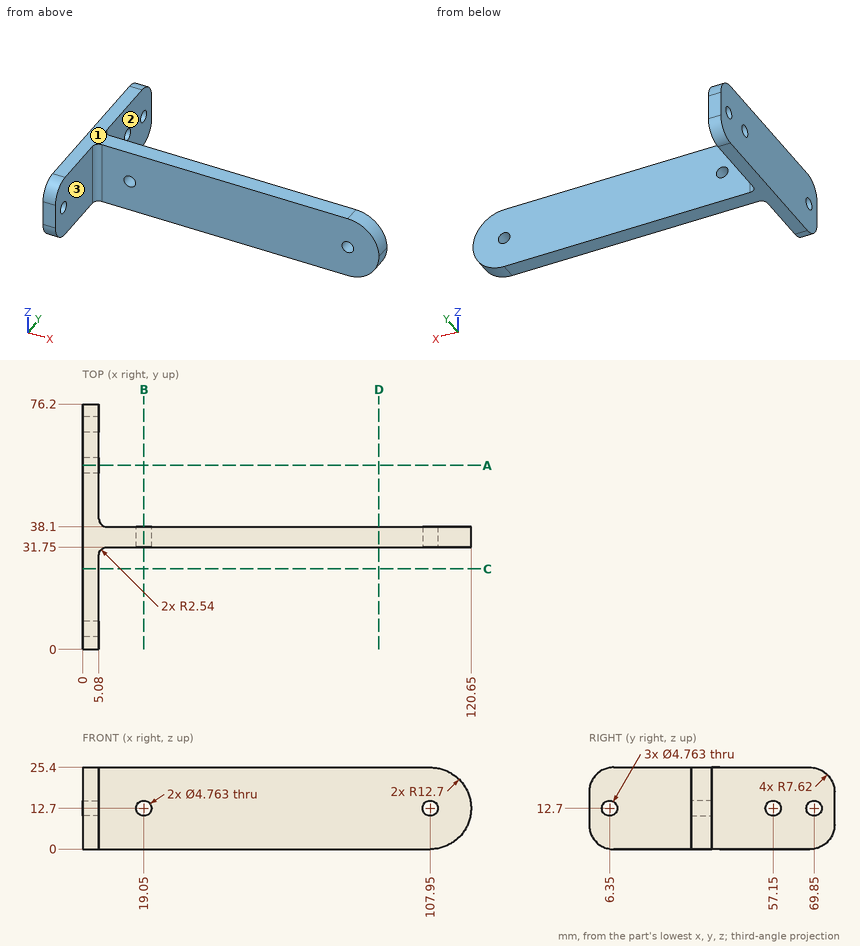
Source: three-view drawing plus pictorial views. Frame: mm from the lowest corner of the part. A direction names the side the tool comes from. Round coordinates to 2 decimals unless told otherwise and drop trailing zeros. Loops run counter-clockwise (first coordinate to the right, second up) from the corner with the lowest first, then second, coordinate; pieces in that order, holes last. Notation, with made-up numbers: (52, -4.5) - (105, -4.5) arc R33 ccw to (105, 26.5) - close; hole circle Ø2 at (-29.5, 5.25). An arc over 180 degrees is marked (long way). Write each question's results on one line, items separated by ' | '. Start each with the question number.
1) Access query for the marked faces 1, 2 and 3. Directions: +Z, -Z, +X, -X, +Y, -Y. A direction counts if a zero-diameter tool reaches every point of the face in a straight line with its end or side. Return the directions, or none.
2) First-contact query: P1, Ø8, axis at x = 84, z = 13, coming from the +Y side; P2, Ø12, axis at y = 30.5, z = 5.5, coming from the +X side; P3, Ø5.5, axis at y = 57.15, z = 12.7, coming from the +X side; P4, Ø6, axis at y = 6.35, z = 12.7, coming from the -X side. Flat tips, straight axial feed; report the tip coordinate or a pass-through.
3) Cut plane D-D on x = 92. Return loops of the section in (y, z), then the cut area to 3 significant figures.
4) Cut plane B-B on x = 19.05. Return loops of the section in (y, z).
5) Line query: probe 1 along Y at (x, z) = (2.25, 12.7); probe 2 along X at (y, z) = (33.25, 12.7); probe 3 along X at (y, z) = (4, 19.5). Output: solid intervals per line, ascending. Write a range as [from, to].
6) Cut plane C-C on y = 25. Return loops of the section in (x, z), then the cut area to 3 significant figures.
7) Cut plane A-A on y = 57.15. Return loops of the section in (x, z).
Verdict:
1) face 1: +Z, +X, -X, +Y, -Y | face 2: +Z, -Z, +X, +Y | face 3: +Z, -Z, +X, -Y
2) P1: stops at y = 38.1 | P2: stops at x = 120.58 | P3: stops at x = 5.08 | P4: stops at x = 0
3) outline: (31.75, 0) - (38.1, 0) - (38.1, 25.4) - (31.75, 25.4) - close | area: 161 mm2
4) outline: (31.75, 0) - (38.1, 0) - (38.1, 10.32) - (31.75, 10.32) - close; (31.75, 15.08) - (38.1, 15.08) - (38.1, 25.4) - (31.75, 25.4) - close
5) probe 1: y = [0, 3.97], [8.73, 54.77], [59.53, 67.47], [72.23, 76.2] | probe 2: x = [0, 16.67], [21.43, 105.57], [110.33, 120.65] | probe 3: x = [0, 5.08]
6) outline: (0, 0) - (5.08, 0) - (5.08, 25.4) - (0, 25.4) - close | area: 129 mm2
7) outline: (0, 0) - (5.08, 0) - (5.08, 10.32) - (0, 10.32) - close; (0, 15.08) - (5.08, 15.08) - (5.08, 25.4) - (0, 25.4) - close
